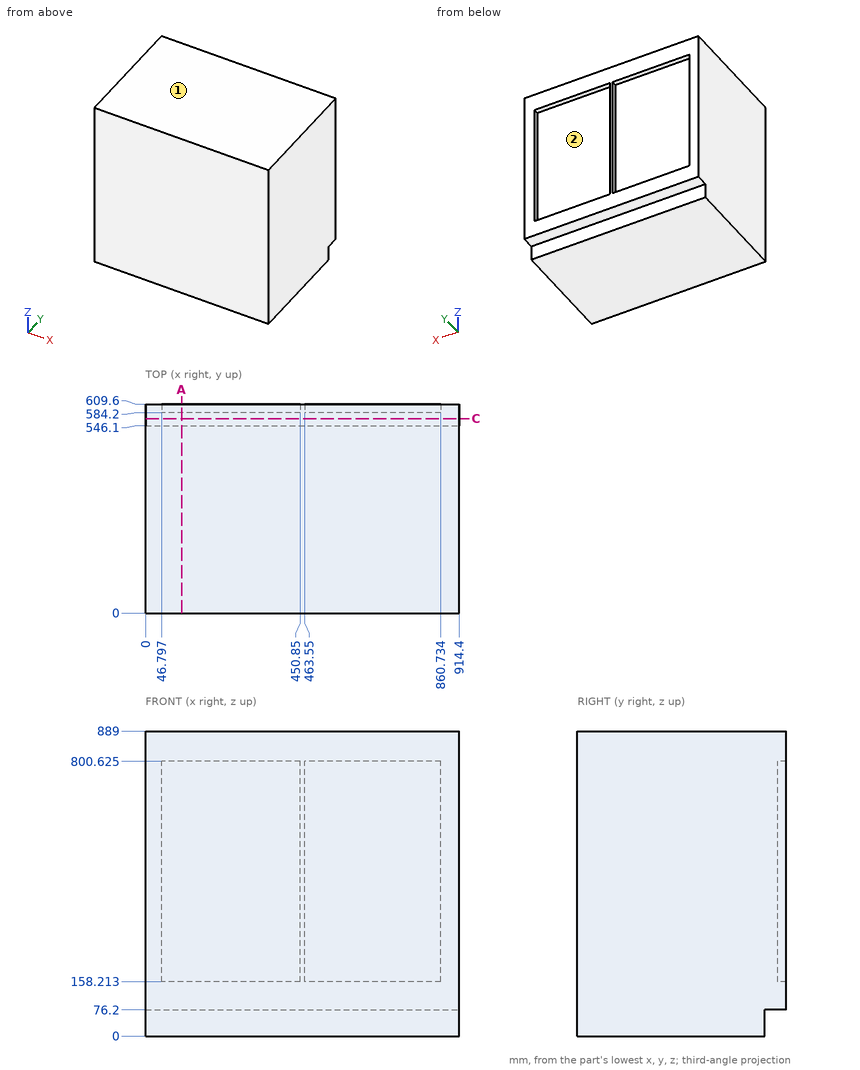
The figure shows three views and two pictorial views of one solid part (mm, origin at its lowest corner). Answer the questions. A direction names the side the tool comes from. Coordinates: 2 decimals unless noted, no trailing zeros. Order: outer loops, then holes, each group sorted by start corner. A loop starts at its lowest first (then second) coordinate and runs counter-clockwise, first axis right, second up.
Q1. A cutting plane is placed at A-A, the plane x = 105. Write down the section's boundary in (y, z) (1 decimal).
Q2. Consider line 1 (Y direction, x = 132, z = 749); line 2 (Z direction, x = 438, y = 575). Determine where each line is inside the solid, lowest interval first.
Q3. A cutting plane is placed at C-C, the plane y = 567. Write down the section's boundary in (x, z).
Q4. Given P1, Ø5, axis at x = 728.5, z = 210.5, coming from the +Y side; P2, Ø12.5, axis at x = 571.5, y = 602.5, coming from the -Z side, each flat-ended and moving along its own axis, determine where each tip first touches the part or whether it passes through.
Q5. Which of the six approach directions +Z, -Z, +X, -X, +Y, -Y give full straight-line access (tool end or side, diameter ignored) to the marked faces 1 and 2?
Answers follow:
1. outline: (0, 0) - (546.1, 0) - (546.1, 76.2) - (609.6, 76.2) - (609.6, 158.2) - (584.2, 158.2) - (584.2, 800.6) - (609.6, 800.6) - (609.6, 889) - (0, 889) - close
2. line 1: y = 0 to 584.2
2. line 2: z = 76.2 to 889
3. outline: (0, 76.2) - (914.4, 76.2) - (914.4, 889) - (0, 889) - close
4. P1: stops at y = 584.2
4. P2: stops at z = 76.2
5. face 1: +Z, +X, -X, +Y, -Y
5. face 2: +Y
